Autodesk Inventor part; units mm, degrees
ref_plane "bf_2_XY" through (0, 0, 0) normal (1, 0, 0) x (0, 0, -1)
ref_plane "bf_2_YZ" through (0, 0, 0) normal (0, 0, -1) x (0, 1, 0)
ref_plane "bf_2_ZX" through (0, 0, 0) normal (0, 1, 0) x (1, 0, 0)
sketch "Sketch_1" plane through (0, 0, 0) normal (0, 0, 1) x (1, 0, 0)
  line L0 (50, 0) -> (-50, 0)
  arc A0 (-4.5, 7.8) -> (-4.2, 7.5) centre (-4.2, 7.8) ccw
  line L1 (-4.2, 7.5) -> (4.2, 7.5)
  arc A1 (4.2, 7.5) -> (4.5, 7.8) centre (4.2, 7.8) ccw
  line L2 (4.5, 7.8) -> (4.5, 15.7)
  arc A2 (4.5, 15.7) -> (4.2, 16) centre (4.2, 15.7) ccw
  line L3 (4.2, 16) -> (-4.2, 16)
  arc A3 (-4.2, 16) -> (-4.5, 15.7) centre (-4.2, 15.7) ccw
  line L4 (-4.5, 15.7) -> (-4.5, 7.8)
revolve "Revolution1" add sketch "Sketch_1" angle 360 about axis through (50, 0, 0) along (1, 0, 0)
sketch "Sketch_2" plane through (0, 0, 0) normal (0, 0, 1) x (1, 0, 0)
  line L0 (50, 0) -> (-50, 0)
  line L1 (-6.3, 13.25) -> (-6.3, 7.5)
  line L2 (-6.3, 7.5) -> (-4.5, 7.5)
  line L3 (-4.5, 7.5) -> (-4.5, 10.2)
  line L4 (-4.5, 10.2) -> (-4.48, 10.2)
  line L5 (-4.48, 10.2) -> (-4.48, 12)
  line L6 (-4.48, 12) -> (-4.3, 12)
  line L7 (-4.3, 12) -> (-4.3, 13.25)
  line L8 (-4.3, 13.25) -> (-6.3, 13.25)
revolve "Revolution2" cut sketch "Sketch_2" angle 360 about axis through (50, 0, 0) along (1, 0, 0)
sketch "Sketch_3" plane through (0, 0, 0) normal (0, 0, 1) x (1, 0, 0)
  line L0 (50, 0) -> (-50, 0)
  line L1 (4.3, 12) -> (4.48, 12)
  line L2 (4.48, 12) -> (4.48, 10.2)
  line L3 (4.48, 10.2) -> (4.5, 10.2)
  line L4 (4.5, 10.2) -> (4.5, 7.5)
  line L5 (4.5, 7.5) -> (6.3, 7.5)
  line L6 (6.3, 7.5) -> (6.3, 13.25)
  line L7 (6.3, 13.25) -> (4.3, 13.25)
  line L8 (4.3, 13.25) -> (4.3, 12)
revolve "Revolution3" cut sketch "Sketch_3" angle 360 about axis through (50, 0, 0) along (1, 0, 0)
ref_plane "bf_2_XY" through (0, 0, 0) normal (1, 0, 0) x (0, 0, -1)
ref_plane "bf_2_YZ" through (0, 0, 0) normal (0, 0, -1) x (0, 1, 0)
ref_plane "bf_2_ZX" through (0, 0, 0) normal (0, 1, 0) x (1, 0, 0)
properties part number "BF 15 Part2"
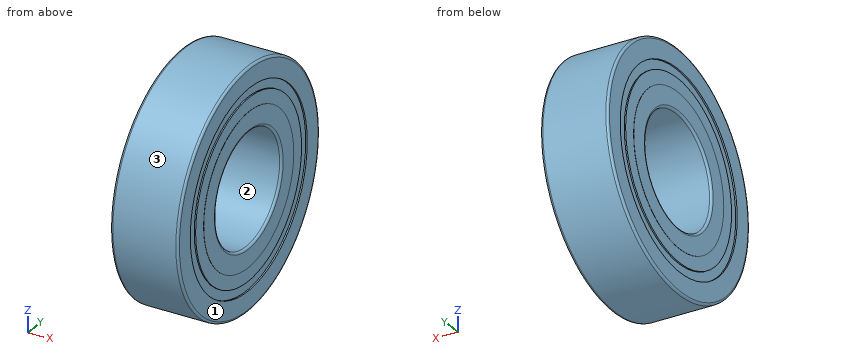
Can you work these out from the model? Positions are in its coordinate system, mm. Face numbers are marked on the shaded views. Coordinates: 2 decimals unless noted, no trailing zeros. Loops run counter-clockwise (first coordinate to the right, second up) from the corner with the lowest first, then second, coordinate; pieces in that order, holes last. Notation, with made-up numbers: (51.5, 85.5) - (88.5, 85.5) arc R23 ccw to (88.5, 97.5) - close; hole circle Ø11 at (-9, 87). An arc over 180 degrees is marked (long way). Answer as CSV lines item,"result". Start each with the question number.
1) For pin 1 (3 mm diameter, centred on x = -1, y = 8, fed in from +Z); pin 2 (6 mm diameter, centred on y = 6, z = 9, fed in from +X); pin 3 (8 mm diameter, centred on y = -2, z = 0, fed in from -X); pin 4 (3 mm diameter, centred on x = 3, y = 9.5, fed in from +Z), each with a flat end and sliding along its axis, tell me the tip position at first contact or that it passes through.
2) Suppose I cut it at A-A (x = 0.5). Please give me the cut outline in (y, z), plus the area to 3 significant figures.
3) Thinking about a two-plate mould opening in Y: for the marked faces 1, 2 and 3, which applies, pulls with the +Y half, pulls with the -Y half, needs draft (parallel to the pull), parting line crosses it, or undercut?
4) I need wall thicknesses on line 1 (Z direction, x = -0.25, y = 0); line 2 (Z direction, x = -4.4, y = 0); line 3 (X direction, y = -8, z = 10). Which ranges of each line are inside material? Lowest first, please. Write a range as from..to.
Check result:
1,pin 1,"stops at z = 14.62"
1,pin 2,"stops at x = 4.5"
1,pin 3,"passes through"
1,pin 4,"stops at z = 13.86"
2,outline,"circle Ø32 at (0, 0); hole circle Ø15 at (0, 0)"
2,area,"628 mm²"
3,face 1,"needs draft"
3,face 2,"undercut"
3,face 3,"parting line crosses it"
4,line 1,"z = -16..-7.5, 7.5..16"
4,line 2,"z = -15.92..-13.25, -12..-7.58, 7.58..12, 13.25..15.92"
4,line 3,"x = -4.3..4.3"
